Here's how the part is built. I have some questions about the finished solid (model axes, mm). Face numbers are marked on the shaded views. A direction names the side the tool comes from. Give positions to 0.01 mm unless a question says otherwise; leave off trailing zeros. Write each loop counter-clockwise with the first axis right and the second up, starting at its lowest first coordinate (ties: lowest second). Pieces come first, ordered by that corner, then holes. Notation, with made-up numbers: M 42.5,75.25 L 67.5,75.25 A13 ccw 67.5,93.25 Z; hole C 21,22.5 d3. An arc over 180 degrees is marked long. Answer as CSV lines item,"result". Start each with the question number.
Q1. For pin 1 (1 mm diameter, centred on y = 12.5, z = 14.5, fed in from +X); pin 2 (10 mm diameter, centred on x = 5, y = 15, fed in from -Z); pin 3 (10 mm diameter, centred on y = -5.5, z = -11.5, fed in from -X), each with a flat end and sliding along its axis, tell me the tip position at first contact or that it passes through.
Q2. Suppose I cut it at C-C (z = -11). Write out the boundary of the cut face in (x, y).
Q3. On a 3-axis mill with a long thin cutter (end or side, diameter ignored), from which of +Z, -Z, +X, -X, +Y, -Y can I reach the whole of each face in a straight line? I mean the marked faces 1 and 2. Say none if no direction works.
Q4. Suppose I cut it at A-A (y = 0). Write out the boundary of the cut face in (x, z), then the cut area to 3 significant figures.
Q5. If I drill on line 1 along Z through (x, y) = (10.5, 15.5); line 2 along Z through (x, y) = (5.5, -5.5); line 3 along Y through (x, z) = (17.5, 20), over which ranges is the centre line in solid material (lowest first)?
Q6. Suppose I cut it at D-D (x = -6). Write out the boundary of the cut face in (y, z), then the cut area to 3 significant figures.
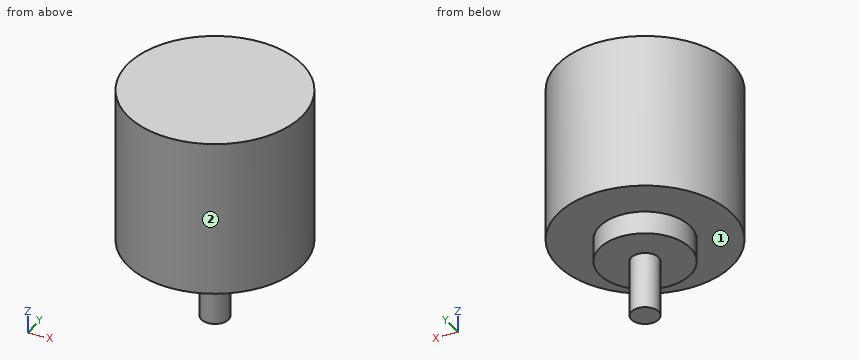
```python
from build123d import *

# Parameters (mm, degrees)
SKETCH1_R           = 19.25
SKETCH1_R_2         = 10
SKETCH1_R_3         = 3
BOSS_EXTRUDE1_DEPTH = 34.5
SKETCH1_3_R         = 10
SKETCH1_3_R_2       = 3
BOSS_EXTRUDE2_DEPTH = 5
SKETCH1_4_R         = 3
BOSS_EXTRUDE3_DEPTH = 17.5


with BuildPart() as part:
    # Sketch1 → Boss-Extrude1 (new body)
    # profile 1 of 3: a face of its own
    with BuildSketch(Plane.XY):
        Circle(SKETCH1_R)
        Circle(SKETCH1_R_2, mode=Mode.SUBTRACT)
    # profile 2 of 3: a face of its own
    with BuildSketch(Plane.XY):
        Circle(SKETCH1_R_2)
        Circle(SKETCH1_R_3, mode=Mode.SUBTRACT)
    # profile 3 of 3: a face of its own
    with BuildSketch(Plane.XY):
        Circle(SKETCH1_R_3)
    extrude(amount=BOSS_EXTRUDE1_DEPTH)

    # Sketch1_3 → Boss-Extrude2 (add)
    with BuildSketch(Plane.XY):
        Circle(SKETCH1_3_R)
        Circle(SKETCH1_3_R_2, mode=Mode.SUBTRACT)
    extrude(amount=-BOSS_EXTRUDE2_DEPTH)

    # Sketch1_4 → Boss-Extrude3 (add)
    with BuildSketch(Plane.XY):
        Circle(SKETCH1_4_R)
    extrude(amount=-BOSS_EXTRUDE3_DEPTH)


solid = part.part
```
Resolved:
1,pin 1,"x = 15.05"
1,pin 2,"z = 0"
1,pin 3,"x = -2.96"
2,outline,"C 0,0 d6"
3,face 1,"-Z"
3,face 2,"+Z, -Z"
4,outline,"M -19.25,0 L -10,0 L -10,-5 L -3,-5 L -3,-17.5 L 3,-17.5 L 3,-5 L 10,-5 L 10,0 L 19.25,0 L 19.25,34.5 L -19.25,34.5 Z"
4,area,"1,500 mm^2"
5,line 1,"0 to 34.5"
5,line 2,"-5 to 34.5"
5,line 3,"-8.02 to 8.02"
6,outline,"M -18.29,0 L -8,0 L -8,-5 L 8,-5 L 8,0 L 18.29,0 L 18.29,34.5 L -18.29,34.5 Z"
6,area,"1,340 mm^2"
